Geometry: see drawing. Coordinates: mm, zero at the bounding-box minimum. Give positions to 0.01 mm unless a question says otherwise; leave off trailing zeros. Loops run counter-clockwise (first coordinate to the right, second up) from the corner with the lowest first, then second, coordinate; pieces in that order, holes last. Notation, with made-up numbers: (20, 21) -> (73, 21) arc R17 cw to (73, 41) -> close; hole circle Ø2 at (55, 8.25). An arc over 180 degrees is marked (long way). One line per question, with ' | ' between items.
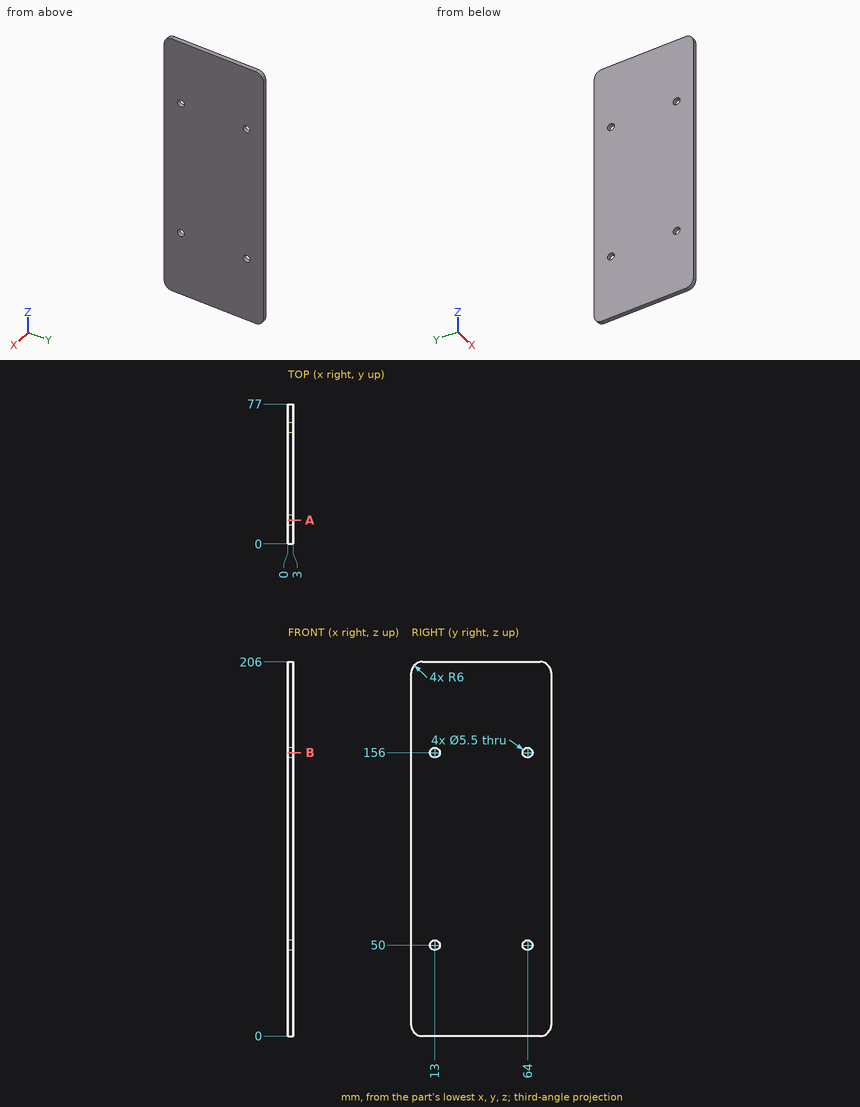
1. Section query A-A (y = 13). Output: boundary loops of the cut face in (x, z).
Determined:
outline: (0, 0) -> (3, 0) -> (3, 47.25) -> (0, 47.25) -> close; (0, 52.75) -> (3, 52.75) -> (3, 153.25) -> (0, 153.25) -> close; (0, 158.75) -> (3, 158.75) -> (3, 206) -> (0, 206) -> close
2. Section query B-B (z = 156). Output: boundary loops of the cut face in (x, y).
Determined:
outline: (0, 0) -> (3, 0) -> (3, 10.25) -> (0, 10.25) -> close; (0, 15.75) -> (3, 15.75) -> (3, 61.25) -> (0, 61.25) -> close; (0, 66.75) -> (3, 66.75) -> (3, 77) -> (0, 77) -> close
3. Ray query, line 1 along Z through (x, y) = (1.8, 64); line 2 along Z through (x, y) = (1.15, 65.5); line 3 along Z through (x, y) = (0.35, 5). Return the intervals inside material, ascending. Write a range as from..to.
Determined:
line 1: z = 0..47.25, 52.75..153.25, 158.75..206 | line 2: z = 0..47.7, 52.3..153.7, 158.3..206 | line 3: z = 0.08..205.92
